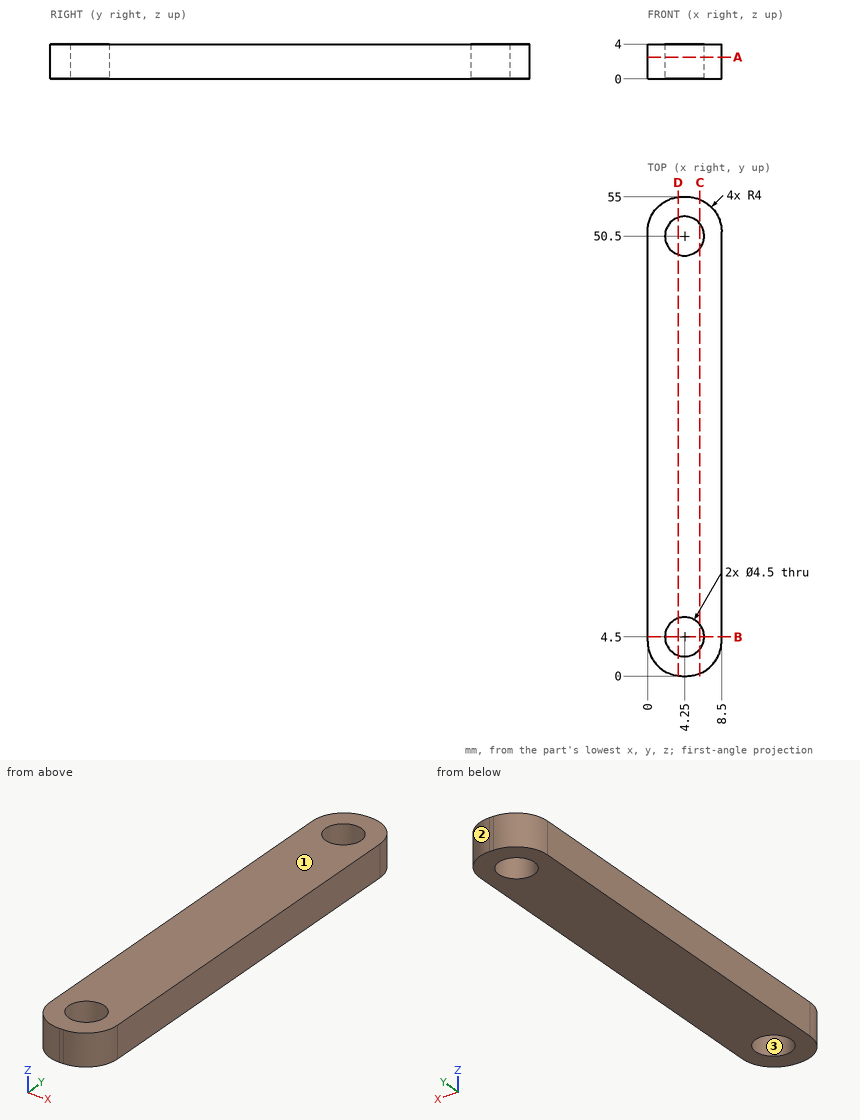
Could you check a few things on this drawing? It's one solid part, dimensions in mm from its lowest x, y, z. Coordinates: 2 decimals unless noted, no trailing zeros. Order: outer loops, then holes, each group sorted by start corner. A loop starts at its lowest first (then second) coordinate and runs counter-clockwise, first axis right, second up. Notation, with made-up numbers: (75, -16) - (109, -16) arc R23 cw to (109, -8) - close; hole circle Ø4 at (-38.75, 52.5). An arc over 180 degrees is marked (long way). Answer as a JSON object with one key per item and string values. Group by question number.
Q1. Imagine slicing it at D-D (x = 3.5). Please give me the cut outline in (y, z).
Q2. We'd pull the mould along X, two halves only. Please class the marked faces 1, 2 and 3: +X half, -X half, draft (parallel to the pull), parting line (faces both ways), or undercut.
Q3. Imagine slicing it at C-C (x = 6). Please give me the cut outline in (y, z).
Q4. Imagine slicing it at A-A (z = 2.5). Please give me the cut outline in (x, y).
Q5. Will this pin go through, and if not, where does the flat tip stop? P1, Ø1.5, axis at x = 1.5, z = 3.5, coming from the -Y side.
Q6. I need wall thicknesses on line 1 (Y direction, x = 4.25, z = 1.75); line 2 (Y direction, x = 3.25, z = 3); line 3 (Y direction, x = 1.5, z = 2.7). Which ranges of each line are inside material? Lowest first, please. Write a range as from..to.
Q7. Imagine slicing it at B-B (y = 4.5). Please give me the cut outline in (x, z).
Determined:
{
 "1": {"outline": "(0.03, 0) - (2.38, 0) - (2.38, 4) - (0.03, 4) - close; (6.62, 0) - (48.38, 0) - (48.38, 4) - (6.62, 4) - close; (52.62, 0) - (54.97, 0) - (54.97, 4) - (52.62, 4) - close"},
 "2": {"face 1": "draft", "face 2": "+X half", "face 3": "undercut"},
 "3": {"outline": "(0.29, 0) - (3.09, 0) - (3.09, 4) - (0.29, 4) - close; (5.91, 0) - (49.09, 0) - (49.09, 4) - (5.91, 4) - close; (51.91, 0) - (54.71, 0) - (54.71, 4) - (51.91, 4) - close"},
 "4": {"outline": "(0, 4) arc R4 ccw to (4, 0) - (4.5, 0) arc R4 ccw to (8.5, 4) - (8.5, 51) arc R4 ccw to (4.5, 55) - (4, 55) arc R4 ccw to (0, 51) - close; hole circle Ø4.5 at (4.25, 4.5); hole circle Ø4.5 at (4.25, 50.5)"},
 "5": {"P1": "stops at y = 0.4"},
 "6": {"line 1": "y = 0..2.25, 6.75..48.25, 52.75..55", "line 2": "y = 0.07..2.48, 6.52..48.48, 52.52..54.93", "line 3": "y = 0.88..54.12"},
 "7": {"outline": "(0, 0) - (2, 0) - (2, 4) - (0, 4) - close; (6.5, 0) - (8.5, 0) - (8.5, 4) - (6.5, 4) - close"}
}
